Autodesk Inventor part; units mm, degrees
ref_plane "YZ Plane" through (0, 0, 0) normal (1, 0, 0) x (0, 1, 0)
ref_plane "XZ Plane" through (0, 0, 0) normal (0, 1, 0) x (-1, 0, 0)
ref_plane "XY Plane" through (0, 0, 0) normal (0, 0, 1) x (1, 0, 0)
sketch "Sketch1" plane through (0, 0, 0) normal (0, 0, 1) x (1, 0, 0)
  line L0 (-21.2139, 7.4194) -> (14.3461, 7.4194)
  line L1 (14.3461, 7.4194) -> (14.3461, -15.1866)
  line L2 (14.3461, -15.1866) -> (-21.2139, -15.1866)
  line L3 (-21.2139, -15.1866) -> (-21.2139, 7.4194)
  point P0 (0, 0)
  dimension "d0" = 22.606
  dimension "d1" = 35.56
extrude "Extrusion1" add sketch "Sketch1" along normal blind 3.81
sketch "Sketch2" plane through (0, 0, 3.81) normal (0, 0, 1) x (1, 0, 0)
  line L0 (14.3461, 7.4194) -> (-21.2139, 7.4194)
  line L1 (-21.2139, -15.1866) -> (14.3461, -15.1866)
  line L2 (14.3461, -15.1866) -> (14.3461, 7.4194)
  line L3 (-21.2139, 7.4194) -> (-21.2139, -15.1866)
  line L4 (5.2021, -2.9946) -> (5.2021, -4.7726)
  line L5 (-12.0699, -4.7726) -> (-12.0699, -2.9946)
  line L6 (5.2021, -4.7726) -> (2.8536, -4.7726)
  line L7 (-9.7213, -4.7726) -> (-12.0699, -4.7726)
  line L8 (-12.0699, -2.9946) -> (-9.7213, -2.9946)
  line L9 (2.8536, -2.9946) -> (5.2021, -2.9946)
  arc A0 (-9.7213, -4.7726) -> (2.8536, -4.7726) centre (-3.4339, -3.8836) ccw
  arc A1 (2.8536, -2.9946) -> (-9.7213, -2.9946) centre (-3.4339, -3.8836) ccw
  point P0 (0, 0)
  dimension "d5" = 11.303
  dimension "d6" = 11.303
  dimension "d7" = 17.78
  dimension "d8" = 17.78
  dimension "d9" = 17.272
  dimension "d10" = 1.778
  dimension "d13" = 9.144
  dimension "d14" = 9.144
extrude "Extrusion2" add sketch "Sketch2" along normal blind 22.86 contours L4 L6 A0 L7 L5 L8 A1 L9
sketch "Sketch3" plane through (0, 0, 26.67) normal (0, 0, 1) x (1, 0, 0)
  line L0 (-7.5614, -0.5816) -> (0.6936, -0.5816)
  line L1 (0.6936, -0.5816) -> (0.6936, -7.1856)
  line L2 (0.6936, -7.1856) -> (-7.5614, -7.1856)
  line L3 (-7.5614, -7.1856) -> (-7.5614, -0.5816)
  line L4 (-12.0699, -2.9946) -> (-12.0699, -4.7726)
  line L5 (5.2021, -4.7726) -> (5.2021, -2.9946)
  arc A0 (2.8536, -2.9946) -> (-9.7213, -2.9946) centre (-3.4339, -3.8836) ccw
  arc A1 (-9.7213, -4.7726) -> (2.8536, -4.7726) centre (-3.4339, -3.8836) ccw
  point P0 (0, 0)
  point P1 (-12.0699, -3.8836)
  point P2 (5.2021, -3.8836)
  point P3 (-3.4339, 2.4664)
  point P4 (-3.4339, -10.2336)
  dimension "d17" = 8.255
  dimension "d18" = 6.604
  dimension "d19" = 4.5085
  dimension "d20" = 4.5085
  dimension "d21" = 3.048
  dimension "d22" = 3.048
extrude "Extrusion3" cut sketch "Sketch3" against normal blind 22.86
sketch "Sketch4" plane through (0, 0, 0) normal (0, 0, -1) x (-1, 0, 0)
  line L0 (1.2749, 4.4984) -> (5.5929, 4.4984)
  line L1 (5.5929, 4.4984) -> (5.5929, -12.2656)
  line L2 (5.5929, -12.2656) -> (1.2749, -12.2656)
  line L3 (1.2749, -12.2656) -> (1.2749, 4.4984)
  line L4 (-14.3461, 7.4194) -> (21.2139, 7.4194)
  line L5 (21.2139, -15.1866) -> (-14.3461, -15.1866)
  line L6 (21.2139, 7.4194) -> (21.2139, -15.1866)
  line L7 (-14.3461, -15.1866) -> (-14.3461, 7.4194)
  point P0 (0, 0)
  point P1 (21.2139, -3.8836)
  dimension "d25" = 4.318
  dimension "d26" = 16.764
  dimension "d27" = 2.921
  dimension "d28" = 2.921
  dimension "d29" = 15.621
  dimension "d30" = 15.621
extrude "Extrusion4" add sketch "Sketch4" along normal blind 5.08 contours L0 L1 L2 L3
fillet "Fillet1" radius 1.5875 2 edges at (-5.5929, -3.8836, -5.08) (-1.2749, -3.8836, -5.08)
fillet "Fillet2" radius 0.8255 4 edges at (-12.0699, -4.7726, 15.24) (-12.0699, -2.9946, 15.24) (5.2021, -4.7726, 15.24) (5.2021, -2.9946, 15.24)
sketch "Sketch5" plane through (0, 0, 0) normal (0, 0, -1) x (-1, 0, 0)
  line L0 (6.4184, -8.3286) -> (6.4184, 0.5614)
  line L1 (6.4184, 0.5614) -> (9.5934, -3.8836)
  line L2 (9.5934, -3.8836) -> (6.4184, -8.3286)
  line L3 (0.4494, -8.3286) -> (0.4494, 0.5614)
  line L4 (0.4494, 0.5614) -> (-2.7256, -3.8836)
  line L5 (-2.7256, -3.8836) -> (0.4494, -8.3286)
  line L6 (5.5929, -12.2656) -> (5.5929, 4.4984)
  line L7 (1.2749, 4.4984) -> (1.2749, -12.2656)
  line L8 (21.2139, -15.1866) -> (-14.3461, -15.1866)
  line L9 (-14.3461, 7.4194) -> (21.2139, 7.4194)
  point P0 (0, 0)
  dimension "d35" = 3.175
  dimension "d36" = 8.89
  dimension "d37" = 0.8255
  dimension "d38" = 0.8255
  dimension "d39" = 6.858
  dimension "d40" = 6.858
  dimension "d41" = 6.858
  dimension "d42" = 6.858
  dimension "d43" = 4.445
  dimension "d44" = 4.445
  dimension "d45" = 4.445
extrude "Extrusion5" add sketch "Sketch5" along normal blind 1.7145
fillet "Fillet3" radius 1.5875 4 edges at (14.3461, 7.4194, 1.905) (14.3461, -15.1866, 1.905) (-21.2139, -15.1866, 1.905) (-21.2139, 7.4194, 1.905)
properties part number "power_switch"
Design review of the part built by this model. Coordinates are the model's own, in mm. A direction names the side the tool comes from. Coordinates: 2 decimals unless noted, no trailing zeros. Order: outer loops, then holes, each group sorted by start corner. A loop starts at its lowest first (then second) coordinate and runs counter-clockwise, first axis right, second up. Notation, with made-up numbers: (-3.5, 22) -> (52.5, 22) arc R23 ccw to (52.5, 30) -> close; hole circle Ø9 at (61.5, -9.75). An arc over 180 degrees is marked (long way). One line per item, written item: value. Start each with the question number.
Q1. Take a section at A-A, the plane z = 22.5. State the section outline as (x, y) points, then the cut area to 3 significant figures.
Q2. For probe 1 along Y at (x, z) = (-2, 14); probe 2 along Z at (x, y) = (12, -10.25); probe 3 along X at (y, z) = (-5.5, 21), list the stretches that pass through material, from the lowest coordinate up.
Q3. Mouldability with a two-part tool opening along Y and no side actions: class faces 1 (the flat face through (-3, 4.498, -3)), 2 (the flat face through (-7.561, -4, 15)), 3 (the cylindrical face through (13.9, -14.7, 1.9)) as pulls with the +Y half, pulls with the -Y half, needs draft (parallel to the pull), parting line crosses it, or undercut.
Q4. Take a section at B-B, the plane y = 5.25. State the section outline as (x, z) points.
Q5. Tool access review of faces 4 (the flat face through (-3, -4, 3.81)), 5 (the flat face through (-8, -4, -1.714)), 6 (the cylindrical face through (-3.561, 2.465, 15.08)), 7 (the cylindrical face through (4.95, -4.54, 15.4)): name each direction out of +Z, -Z, +X, -X, +Y, -Y from which nothing blocks a thin tool from reaching the whole face with its end or side.
Q6. Take a section at C-C, the plane x = -8.5. State the section outline as (y, z) points, then the cut area to 3 significant figures.
Q7. Take a section at D-D, the plane x = 10. State the section outline as (y, z) points.
Q8. Insertion check: pin 1 Ø1 at (x, y) = (-12, -1) entering from +Z; pin 2 Ø3 at (y, z) = (-6.5, -1) entering from +X; pin 3 Ø4 at (x, z) = (-1.5, 19) entering from -Y; pin 4 Ø4 at (y, z) = (-6.5, -2.5) entering from -X. Each pin has a flat end and moves straight along its axis. Give the tip position at first contact, or say it passes through.
Values follow:
1. outline: (-12.07, -3.95) arc R0.83 ccw to (-11.24, -4.77) -> (-9.72, -4.77) arc R6.35 ccw to (2.85, -4.77) -> (4.38, -4.77) arc R0.83 ccw to (5.2, -3.95) -> (5.2, -3.82) arc R0.83 ccw to (4.38, -2.99) -> (2.85, -2.99) arc R6.35 ccw to (-9.72, -2.99) -> (-11.24, -2.99) arc R0.83 ccw to (-12.07, -3.82) -> close; hole (-7.56, -7.19) -> (0.69, -7.19) -> (0.69, -0.58) -> (-7.56, -0.58) -> close
1. area: 79.8 mm2
2. probe 1: y = -10.07 to -7.19, -0.58 to 2.3
2. probe 2: z = 0 to 3.81
2. probe 3: x = -9.57 to -7.56, 0.69 to 2.71
3. face 1: pulls with the +Y half
3. face 2: undercut
3. face 3: pulls with the -Y half
4. outline: (-21.21, 0) -> (14.35, 0) -> (14.35, 3.81) -> (-21.21, 3.81) -> close
5. face 4: +Z
5. face 5: -Z, -X, +Y, -Y
5. face 6: +Z, +Y
5. face 7: +Z, +X, -Y
6. outline: (-15.19, 0) -> (-5.41, 0) -> (-5.41, -1.71) -> (-2.35, -1.71) -> (-2.35, 0) -> (7.42, 0) -> (7.42, 3.81) -> (-0.06, 3.81) -> (-0.06, 26.67) -> (-7.71, 26.67) -> (-7.71, 3.81) -> (-15.19, 3.81) -> close
6. area: 266 mm2
7. outline: (-15.19, 0) -> (7.42, 0) -> (7.42, 3.81) -> (-15.19, 3.81) -> close
8. pin 1: stops at z = 3.81
8. pin 2: stops at x = 14.35
8. pin 3: stops at y = -10.23
8. pin 4: stops at x = -9.04
